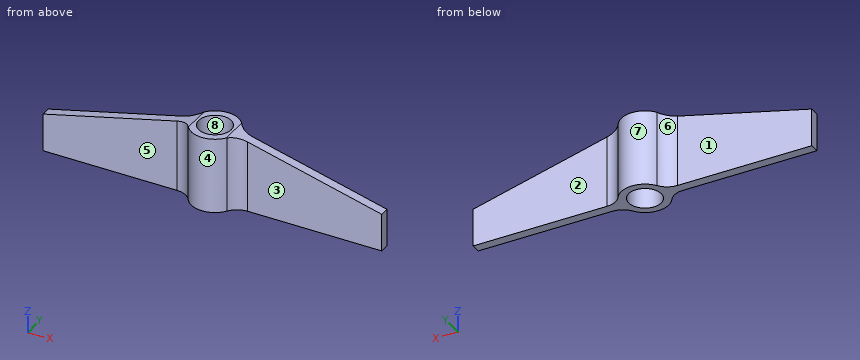
```python
from build123d import *

# Parameters (mm, degrees)
F0_R     = 4.3
F1_DEPTH = 20
F2_R     = 5
F3_SIZE2 = 10
F3_SIZE  = 40


with BuildPart() as f1:
    # F0 (on Top) → F1 (new body)
    with BuildSketch(Plane.XY):
        with BuildLine():
            Line((-45, -1.25), (-6.123724357, -1.25))
            ThreePointArc((-6.123724357, -1.25), (0, -6.25), (6.123724357, -1.25))
            Line((6.123724357, -1.25), (45, -1.25))
            Line((45, -1.25), (45, 1.25))
            Line((45, 1.25), (6.123724357, 1.25))
            ThreePointArc((6.123724357, 1.25), (0, 6.25), (-6.123724357, 1.25))
            Line((-6.123724357, 1.25), (-45, 1.25))
            Line((-45, 1.25), (-45, -1.25))
        make_face()
        Circle(F0_R, mode=Mode.SUBTRACT)
    extrude(amount=F1_DEPTH)

    # F2
    f2_edges = [f1.edges().sort_by_distance(p)[0] for p in [
        (-6.123724, -1.25, 10),
        (6.123724, -1.25, 10),
        (-6.123724, 1.25, 10),
        (6.123724, 1.25, 10),
    ]]
    fillet(f2_edges, radius=F2_R)

    # F3
    f3_edges = [f1.edges().sort_by_distance(p)[0] for p in [
        (-45, 0, 20),
        (45, 0, 20),
    ]]
    f3_side = f1.faces().sort_by_distance((-27.177072, 0.341361, 20))[0]
    chamfer(f3_edges, length=F3_SIZE, length2=F3_SIZE2, reference=f3_side)


solid = f1.part
```
CAD build for the part. Positions are in the model's coordinates, mm. Face numbers are marked on the shaded views. A direction names the side the tool comes from. Give positions to 0.01 mm unless a question says otherwise; leave off trailing zeros. Loops run counter-clockwise (first coordinate to the right, second up) from the corner with the lowest first, then second, coordinate; pieces in that order, holes last. Notation, with made-up numbers: (59.5, -31.5) - (64.5, -31.5) arc R34 cw to (64.5, 1.5) - close; hole circle Ø3 at (79, -37.5). An arc over 180 degrees is marked (long way). Put each result on its own line as item: value.
Q1. Slice it at C-C (x = 0). Give the cut face in (y, z).
Filled in:
outline: (-6.25, 0) - (-4.3, 0) - (-4.3, 20) - (-6.25, 20) - close; (4.3, 0) - (6.25, 0) - (6.25, 20) - (4.3, 20) - close
Q2. Probe line 1 along Y through (x, z) = (0, 13.25); line 2 along Y through (x, z) = (-5, 2); line 3 along Y through (x, z) = (-14, 11). List the from-to ranges inside material, lowest first.
Filled in:
line 1: y = -6.25 to -4.3, 4.3 to 6.25
line 2: y = -3.75 to 3.75
line 3: y = -1.25 to 1.25
Q3. Flat gauge pins, fed straight in: pin 1 (1.5 mm diameter, centred on x = 18.5, y = 0, fed in from +Z); pin 2 (5 mm diameter, centred on x = -26, z = 10.5, fed in from -Y); pin 3 (5.5 mm diameter, centred on x = 25, z = 13.5, fed in from +Y); pin 4 (5 mm diameter, centred on x = 2.5, z = 6, fed in from -Y). Where does each tip first touch, or does it go through?
Filled in:
pin 1: stops at z = 16.81
pin 2: stops at y = -1.25
pin 3: stops at y = 1.25
pin 4: stops at y = -6.25
Q4. Slice it at D-D (z = 15.5). Give the cut face in (x, y).
Filled in:
outline: (-23, -1.25) - (-9.35, -1.25) arc R5 cw to (-5.2, -3.47) arc R6.25 ccw to (5.2, -3.47) arc R5 cw to (9.35, -1.25) - (23, -1.25) - (23, 1.25) - (9.35, 1.25) arc R5 cw to (5.2, 3.47) arc R6.25 ccw to (-5.2, 3.47) arc R5 cw to (-9.35, 1.25) - (-23, 1.25) - close; hole circle Ø8.6 at (0, 0)
Q5. Mould opens along X. For the marked faces 6, 7 and 8 say: pulls with the +X half, pulls with the -X half, needs draft (parallel to the pull), parting line crosses it, or undercut.
Filled in:
face 6: pulls with the -X half
face 7: parting line crosses it
face 8: undercut
Q6. Tool access for the marked faces 1, 2, 3, 4 and 5: list every direction of +Z, -Z, +X, -X, +Y, -Y with a clear straight run to the whole face (end or side of a thin tool).
Filled in:
face 1: +Z, -Z, -X, +Y
face 2: +Z, -Z, +X, +Y
face 3: +Z, -Z, +X, -Y
face 4: +Z, -Z, -Y
face 5: +Z, -Z, -X, -Y
Q7. Slice it at B-B (z = 1.5). Give the cut face in (x, y).
Filled in:
outline: (-45, -1.25) - (-9.35, -1.25) arc R5 cw to (-5.2, -3.47) arc R6.25 ccw to (5.2, -3.47) arc R5 cw to (9.35, -1.25) - (45, -1.25) - (45, 1.25) - (9.35, 1.25) arc R5 cw to (5.2, 3.47) arc R6.25 ccw to (-5.2, 3.47) arc R5 cw to (-9.35, 1.25) - (-45, 1.25) - close; hole circle Ø8.6 at (0, 0)
Q8. Slice it at A-A (y = 0). Give the cut face in (x, z), plus the area to 3 significant figures.
Filled in:
outline: (-45, 0) - (-4.3, 0) - (-4.3, 20) - (-5, 20) - (-45, 10) - close; (4.3, 0) - (45, 0) - (45, 10) - (5, 20) - (4.3, 20) - close
area: 1,230 mm²
